Autodesk Inventor part; units mm, degrees
ref_plane "YZ Plane" through (0, 0, 0) normal (1, 0, 0) x (0, 1, 0)
ref_plane "XZ Plane" through (0, 0, 0) normal (0, 1, 0) x (-1, 0, 0)
ref_plane "XY Plane" through (0, 0, 0) normal (0, 0, 1) x (1, 0, 0)
sketch "Sketch1" plane through (0, 0, 0) normal (0, 1, 0) x (-1, 0, 0)
  line L0 (0, 0) -> (0, -104.6)
  line L1 (0, -104.6) -> (-73.9634, -73.9634)
  line L2 (-73.9634, -73.9634) -> (-104.6, 0)
  line L3 (-104.6, 0) -> (-73.9634, 73.9634)
  line L4 (-73.9634, 73.9634) -> (0, 104.6)
  line L5 (0, 104.6) -> (73.9634, 73.9634)
  line L6 (73.9634, 73.9634) -> (104.6, 0)
  line L7 (104.6, 0) -> (73.9634, -73.9634)
  line L8 (73.9634, -73.9634) -> (0, -104.6)
  line L9 (89.2707, -89.2707) -> (126.2478, 0)
  line L10 (126.2478, 0) -> (89.2707, 89.2707)
  line L11 (89.2707, 89.2707) -> (0, 126.2478)
  line L12 (0, 126.2478) -> (-89.2707, 89.2707)
  line L13 (-89.2707, 89.2707) -> (-126.2478, 0)
  line L14 (-126.2478, 0) -> (-89.2707, -89.2707)
  line L15 (-89.2707, -89.2707) -> (0, -126.2478)
  line L16 (0, -126.2478) -> (89.2707, -89.2707)
  line L17 (0, -104.6) -> (7.6537, -123.0776)
  line L18 (0, -104.6) -> (20, -104.6) construction
  line L19 (73.9634, -73.9634) -> (81.617, -92.441)
  line L20 (73.9634, -73.9634) -> (76.2595, -79.5066)
  line L21 (76.2595, -79.5066) -> (70.7162, -81.8027)
  circle A0 centre (70.7162, -81.8027) radius 1.6
  line L22 (0, -104.6) -> (2.2961, -110.1433)
  line L23 (2.2961, -110.1433) -> (7.8394, -107.8472)
  circle A1 centre (7.8394, -107.8472) radius 1.6
  circle A2 centre (107.8472, -7.8394) radius 1.6
  circle A3 centre (81.8027, -70.7162) radius 1.6
  circle A4 centre (81.8027, 70.7162) radius 1.6
  circle A5 centre (107.8472, 7.8394) radius 1.6
  circle A6 centre (7.8394, 107.8472) radius 1.6
  circle A7 centre (70.7162, 81.8027) radius 1.6
  circle A8 centre (-70.7162, 81.8027) radius 1.6
  circle A9 centre (-7.8394, 107.8472) radius 1.6
  circle A10 centre (-107.8472, 7.8394) radius 1.6
  circle A11 centre (-81.8027, 70.7162) radius 1.6
  circle A12 centre (-81.8027, -70.7162) radius 1.6
  circle A13 centre (-107.8472, -7.8394) radius 1.6
  circle A14 centre (-7.8394, -107.8472) radius 1.6
  circle A15 centre (-70.7162, -81.8027) radius 1.6
  dimension "d0" = 104.6
  dimension "d1" = 20
  dimension "d2" = 67.5
  dimension "d3" = 6
  dimension "d4" = 6
  dimension "d5" = 3.2
  dimension "d6" = 6
  dimension "d7" = 3.2
  dimension "d10" = 360
extrude "Extrusion1" add sketch "Sketch1" along normal blind 6
sketch "Sketch2" plane through (0, 6, 0) normal (0, 1, 0) x (1, 0, 0)
  circle A0 centre (-42.6783, -41.3923) radius 1.25
  circle A1 centre (-71.1016, 20.1286) radius 1.25
  circle A2 centre (9.5684, 59.7961) radius 1.25
  circle A3 centre (50.6037, -21.3711) radius 1.25
  line L0 (27.326, 15.8388) -> (30.0184, 17.162)
  line L1 (30.0184, 17.162) -> (27.8131, 21.6494)
  line L2 (-6.9954, 48.8338) -> (-9.6878, 47.5107)
  line L3 (-9.6878, 47.5107) -> (-7.4825, 43.0233)
  line L4 (25.1207, 20.3262) -> (27.326, 15.8388)
  line L5 (27.8131, 21.6494) -> (25.1207, 20.3262)
  line L6 (-7.4825, 43.0233) -> (-4.7901, 44.3464)
  line L7 (-4.7901, 44.3464) -> (-6.9954, 48.8338)
  line L8 (-12.62, -33.9245) -> (-10.9955, -28.7261)
  line L9 (-10.9955, -28.7261) -> (-27.141, -23.6807)
  line L10 (-27.141, -23.6807) -> (-28.7655, -28.879)
  line L11 (-28.7655, -28.879) -> (-12.62, -33.9245)
  line L12 (-12.62, -33.9245) -> (-27.141, -23.6807) construction
  line L13 (-10.9955, -28.7261) -> (-28.7655, -28.879) construction
  line L14 (-45.832, -38.6971) -> (-42.9662, -37.2994)
  line L15 (-42.9662, -37.2994) -> (-63.3038, 4.3989)
  line L16 (-63.3038, 4.3989) -> (-66.1696, 3.0011)
  line L17 (-66.1696, 3.0011) -> (-45.832, -38.6971)
  line L18 (-45.832, -38.6971) -> (-63.3038, 4.3989) construction
  line L19 (-42.9662, -37.2994) -> (-66.1696, 3.0011) construction
  line L20 (-45.832, -38.6971) -> (-42.6435, -38.6971) construction
  line L21 (-57.8864, 3.7) -> (-59.1996, 6.4006)
  line L22 (-59.1996, 6.4006) -> (-52.2421, 9.7838)
  line L23 (-52.2421, 9.7838) -> (-50.9289, 7.0832)
  line L24 (-50.9289, 7.0832) -> (-57.8864, 3.7)
  line L25 (-64.7367, 19.4057) -> (-67.0188, 24.0494)
  line L26 (-67.0188, 24.0494) -> (-58.9321, 28.0235)
  line L27 (-58.9321, 28.0235) -> (-56.65, 23.3798)
  line L28 (-56.65, 23.3798) -> (-64.7367, 19.4057)
  line L29 (-52.2421, 24.5164) -> (-64.1558, 49.0938)
  line L30 (-64.1558, 49.0938) -> (-52.3886, 54.7979)
  line L31 (-52.3886, 54.7979) -> (-40.4749, 30.2205)
  line L32 (-40.4749, 30.2205) -> (-52.2421, 24.5164)
  line L33 (-29.4108, 46.112) -> (-24.4587, 36.7338)
  line L34 (-24.4587, 36.7338) -> (-14.7376, 41.867)
  line L35 (-14.7376, 41.867) -> (-19.6897, 51.2451)
  line L36 (-19.6897, 51.2451) -> (-29.4108, 46.112)
  circle A4 centre (9.5684, 59.7961) radius 1.75
  circle A5 centre (50.6037, -21.3711) radius 1.75
  circle A6 centre (-42.6783, -41.3923) radius 1.75
  circle A7 centre (-71.1016, 20.1286) radius 1.75
  line L37 (26.8696, 14.5003) -> (31.357, 16.7056)
  line L38 (31.357, 16.7056) -> (28.2696, 22.9879)
  line L39 (28.2696, 22.9879) -> (23.7822, 20.7827)
  line L40 (23.7822, 20.7827) -> (26.8696, 14.5003)
  line L41 (-6.539, 50.1724) -> (-11.0263, 47.9671)
  line L42 (-11.0263, 47.9671) -> (-7.9389, 41.6847)
  line L43 (-7.9389, 41.6847) -> (-3.4516, 43.89)
  line L44 (-3.4516, 43.89) -> (-6.539, 50.1724)
  point P0 (0, 0)
  point P1 (-19.8805, -28.8026)
  point P2 (-54.5679, -17.1491)
  dimension "d14" = 26
  dimension "d15" = 0.5
  dimension "d16" = 0.5
  dimension "d17" = 0.5
  dimension "d18" = 0.5
  dimension "d19" = 1
  dimension "d20" = 1
extrude "Extrusion2" cut sketch "Sketch2" against normal blind 7 contours A0 | A1 | A2 | A3 | L4 L5 L1 L0 | L7 L6 L3 L2 | L11 L10 L9 L8 | L17 L16 L15 L14 | L21 L22 L23 L24 | L25 L26 L27 L28 | L29 L30 L31 L32 | L36 L35 L34 L33 | A4 | A5 | A6 | A7 | L40 L39 L38 L37 | L44 L43 L42 L41
fillet "Fillet1" radius 2 8 edges at (89.2707, 3, 89.2707) (126.2478, 3, 0) (89.2707, 3, -89.2707) (0, 3, -126.2478) (-89.2707, 3, -89.2707) (-126.2478, 3, 0) (-89.2707, 3, 89.2707) (0, 3, 126.2478)
properties part number "Bund"
For this review, take the finished solid that the model builds, in its own axes (mm). A direction names the side the tool comes from. Coordinates: 2 decimals unless noted, no trailing zeros. Loops run counter-clockwise (first coordinate to the right, second up) from the corner with the lowest first, then second, coordinate; pieces in that order, holes last.
1. Add section B-B, the plane y = 2.4. Count the separate pieces of the cut face and the enclosed holes in it, then the cut area to 3 significant figures.
2. For line 1 (Z direction, x = -55.5, y = 5.65); line 2 (X direction, y = 2.25, z = -26); line 3 (X direction, y = 1.6, z = 70), list the stretches that pass through material, from the lowest coordinate up.
3. Add section C-C, the plane z = 100.5. Give the boundary of the cut face in (x, y), then the cut area to 3 significant figures.
4. Add section A-A, the plane z = -101. Give the boundary of the cut face in (x, y), then the cut area to 3 significant figures.
5. Insertion check: P1, Ø3, axis at y = 3.5, z = -40.5, coming from the -X side; P2, Ø2, axis at x = 51, y = 1.5, coming from the -Z side; P3, Ø1.5, axis at y = 3, z = -59.5, coming from the +X side. Each pin has a flat end and moves straight along its axis. Give the tip position at first contact, or say it passes through.
6. Mouldability with a two-part tool opening along X and no side actions: class faces 1 (the flat face through (107.505, 2.958, 45.25)), 2 (the flat face through (2, 6, 2)), 3 (the flat face through (-19.666, 3.042, -39.264)) as +X half, -X half, draft (parallel to the pull), parting line (faces both ways), or undercut.
7. For faces 4 (the flat face through (-44.021, 2.958, -108.014)), 5 (the flat face through (-46.515, 3.042, -42.681)), list the 3-axis set-ups (+Z, -Z, +X, -X, +Y, -Y) from which the entire face can be reached by the end or side of a thin tool; tool diameter is ignored.
Result:
1. separate pieces: 1
1. enclosed holes: 28
1. area: 44,100 mm2
2. line 1: z = -103.26 to -53.29, -31.24 to -8.2, -4.86 to 11.6, 18.87 to 103.26
2. line 2: x = -115.48 to -63.05, -57.94 to -52.96, -49.18 to 115.48
2. line 3: x = -97.25 to -83.23, -80.37 to 80.37, 83.23 to 97.25
3. outline: (-62.16, 0) - (62.16, 0) - (62.16, 6) - (-62.16, 6) - close
3. area: 746 mm2
4. outline: (-60.95, 0) - (60.95, 0) - (60.95, 6) - (-60.95, 6) - close
4. area: 731 mm2
5. P1: stops at x = -110.09
5. P2: stops at z = -105.54
5. P3: stops at x = 101.91
6. face 1: +X half
6. face 2: draft
6. face 3: undercut
7. face 4: -Z, -X, +Y, -Y
7. face 5: +Y, -Y
